from build123d import *

# Parameters (mm, degrees)
SKETCH1_W               = 95.25
SKETCH1_H               = 8.466666667
BOSS_EXTRUDE1_DEPTH     = 38.1
SKETCH2_W               = 6.35
SKETCH2_H               = 127
BOSS_EXTRUDE2_DEPTH     = 38.1
SKETCH3_W               = 88.9
SKETCH3_H               = 8.466666667
BOSS_EXTRUDE3_DEPTH     = 38.1
SKETCH4_R               = 11
CUT_EXTRUDE1_DEPTH      = 149.412147835
SKETCH5_R               = 2.15265
CUT_EXTRUDE2_DEPTH      = 149.412147835
FILLET1_R               = 7.62
BOSS_EXTRUDE4_DEPTH     = 38.1
CUT_EXTRUDE8_REACH      = 172.773
CUT_EXTRUDE8_END_RADIUS = 38.1
FILLET2_R               = 11.688947
FILLET3_R               = 11.688947
FILLET4_R               = 6.35


with BuildPart() as part:
    # Sketch1 → Boss-Extrude1 (new body)
    with BuildSketch(Plane(origin=(0, 0, 0), x_dir=(1, 0, 0), z_dir=(0, 1, 0))):
        with Locations((19.05, 13.758333334)):
            Rectangle(SKETCH1_W, SKETCH1_H)
    extrude(amount=BOSS_EXTRUDE1_DEPTH)

    # Sketch2 → Boss-Extrude2 (add)
    with BuildSketch(Plane(origin=(0, 38.1, 0), x_dir=(1, 0, 0), z_dir=(0, 1, 0))):
        with Locations((63.5, 73.025)):
            Rectangle(SKETCH2_W, SKETCH2_H)
    extrude(amount=-BOSS_EXTRUDE2_DEPTH)

    # Sketch3 → Boss-Extrude3 (add)
    with BuildSketch(Plane(origin=(0, 38.1, 0), x_dir=(1, 0, 0), z_dir=(0, 1, 0))):
        with Locations((15.875, 132.291666667)):
            Rectangle(SKETCH3_W, SKETCH3_H)
    extrude(amount=-BOSS_EXTRUDE3_DEPTH)

    # Sketch4 → Cut-Extrude1 (cut, through all)
    with BuildSketch(Plane(origin=(0, 0, -136.525), x_dir=(-1, 0, 0), z_dir=(0, 0, -1))):
        with Locations((-31.75, 19.05)):
            Circle(SKETCH4_R)
    extrude(amount=-CUT_EXTRUDE1_DEPTH, mode=Mode.SUBTRACT)

    # Sketch5 → Cut-Extrude2 (cut, through all)
    with BuildSketch(Plane(origin=(0, 0, -136.525), x_dir=(-1, 0, 0), z_dir=(0, 0, -1))):
        with Locations((-18.877667779, 26.704865736)):
            Circle(SKETCH5_R)
        with Locations((-19.228536904, 10.833743663)):
            Circle(SKETCH5_R)
        with Locations((-44.622332221, 11.395134264)):
            Circle(SKETCH5_R)
        with Locations((-44.271463096, 27.266256337)):
            Circle(SKETCH5_R)
    extrude(amount=-CUT_EXTRUDE2_DEPTH, mode=Mode.SUBTRACT)

    # Fillet1
    fillet1_edges = [part.edges().sort_by_distance(p)[0] for p in [
        (66.675, 19.05, -136.525),
        (66.675, 19.05, -9.525),
    ]]
    fillet(fillet1_edges, radius=FILLET1_R)

    # Sketch10 → Boss-Extrude4 (add)
    with BuildSketch(Plane(origin=(0, 38.1, 0), x_dir=(1, 0, 0), z_dir=(0, 1, 0))):
        with BuildLine():
            Line((-28.575, 17.991666667), (-28.575, 9.525))
            Line((-28.575, 9.525), (-34.925, 9.525))
            Line((-34.925, 9.525), (-34.925, 25.781))
            Line((-34.925, 25.781), (-5.996027965, 57.15))
            ThreePointArc((-5.996027965, 57.15), (-2.531188929, 73.025), (-5.996027965, 88.9))
            Line((-5.996027965, 88.9), (-34.925, 120.269))
            Line((-34.925, 120.269), (-34.925, 136.525))
            Line((-34.925, 136.525), (-28.575, 136.525))
            Line((-28.575, 136.525), (-28.575, 123.825))
            Line((-28.575, 123.825), (-10.494392478, 104.219375))
            ThreePointArc((-10.494392478, 104.219375), (2.742945437, 73.025), (-10.494392478, 41.830625))
            Line((-10.494392478, 41.830625), (-28.575, 22.225))
            Line((-28.575, 22.225), (-28.575, 17.991666667))
        make_face()
    extrude(amount=-BOSS_EXTRUDE4_DEPTH)

    # Cut-Extrude8: up to this cylinder (the profile starts outside it)
    cut_extrude8_end = Plane(origin=(-40.631188929, 2.695024, -73.025), z_dir=(0, 1, 0)) * Cylinder(CUT_EXTRUDE8_END_RADIUS, 422.746, mode=Mode.PRIVATE)
    # Sketch12 → Cut-Extrude8 (cut, up to the surface)
    with BuildSketch(Plane.ZY.offset(-60.325), mode=Mode.PRIVATE) as cut_extrude8_sk1:
        with BuildLine():
            Line((-79.375, 0), (-66.675, 0))
            ThreePointArc((-66.675, 0), (-73.025, 6.35), (-79.375, 0))
        make_face()
    cut_extrude8_tool1 = extrude(cut_extrude8_sk1.sketch, amount=CUT_EXTRUDE8_REACH, mode=Mode.PRIVATE) - cut_extrude8_end
    add(cut_extrude8_tool1.solids().sort_by_distance((60.325, 2.695024, -73.025))[0], mode=Mode.SUBTRACT)

    # Fillet2
    fillet2_edges = [part.edges().sort_by_distance(p)[0] for p in [
        (-34.925, 19.05, -136.525),
        (-34.925, 19.05, -120.269),
    ]]
    fillet(fillet2_edges, radius=FILLET2_R - 0.0001)  # a hair under: the kernel refuses the full size

    # Fillet3
    fillet3_edges = [part.edges().sort_by_distance(p)[0] for p in [
        (-34.925, 19.05, -25.781),
        (-34.925, 19.05, -9.525),
    ]]
    fillet(fillet3_edges, radius=FILLET3_R - 0.0001)  # a hair under: the kernel refuses the full size

    # Fillet4
    fillet4_edges = [part.edges().sort_by_distance(p)[0] for p in [
        (60.325, 19.05, -17.991666667),
        (60.325, 19.05, -128.058333333),
    ]]
    fillet(fillet4_edges, radius=FILLET4_R)


solid = part.part
Geometry: final body of the model. Coordinates: model frame, mm. A direction names the side the tool comes from. Coordinates: 2 decimals unless noted, no trailing zeros. Loops run counter-clockwise (first coordinate to the right, second up) from the corner with the lowest first, then second, coordinate; pieces in that order, holes last. Notation, with made-up numbers: (28.25, 46) - (33.25, 46) arc R13 cw to (33.25, 65) - close; hole circle Ø10 at (24.25, -13). An arc over 180 degrees is marked (long way). Put each result on its own line as item: value. Start each with the question number.
Q1. Cut plane A-A, the plane x = 31.75. Return loops of the section in (y, z) (3 decimals), and give its area (3 significant figures).
Q2. Line query: line 1 (Z direction, x = 44, y = 20) (3 decimals); line 2 (Z direction, x = -23, y = 29.5) (3 decimals); line 3 (Y direction, x = 31.75, z = -131). Output: solid intervals per line, ascending.
Q3. Set-up query: faces 4 (the flat face through (-28.575, 19, -126)), 5 (the flat face through (-19, 19, -103)), 6 (the cylindrical face through (45.86, 28.72, -132.35)). Return all of +Z, -Z, +X, -X, +Y, -Y with unobstructed straight access to the full face (end or side cutting, diameter ignored); none if empty.
Q4. Pin query (flat end, axial travel): pin 1 Ø1 at (y, z) = (4, -37) entering from -X; pin 2 Ø1.5 at (y, z) = (18, -101) entering from -X. Return the tip coordinate at first contact, or that it passes through.
Q5. Cut plane C-C, the plane z = -84.5. Return loops of the section in (x, y) (1 decimal), and give its area (3 significant figures).
Q6. Pull-direction query (Z, two-part tool) for faces 1 (the cylindrical face through (45.86, 28.72, -13.82)), 2 (the flat face through (12, 19, -128.058)), 3 (the cylindrical face through (64.384, 18.783, -134.352)); classes: released by +Z, released by -Z, zero draft, split by the parting line, or undercut.
Filled sheet:
1. outline: (0, -136.525) - (8.05, -136.525) - (8.05, -128.058) - (0, -128.058) - close; (0, -17.992) - (8.05, -17.992) - (8.05, -9.525) - (0, -9.525) - close; (30.05, -136.525) - (38.1, -136.525) - (38.1, -128.058) - (30.05, -128.058) - close; (30.05, -17.992) - (38.1, -17.992) - (38.1, -9.525) - (30.05, -9.525) - close
1. area: 273 mm²
2. line 1: -136.525 to -128.058, -17.992 to -9.525
2. line 2: -136.525 to -128.058, -117.78 to -107.338, -38.712 to -28.27, -17.992 to -9.525
2. line 3: 0 to 8.05, 30.05 to 38.1
3. face 4: +Y, -Y
3. face 5: -X, +Y, -Y
3. face 6: +Z, -Z
4. pin 1: x = -25.04
4. pin 2: x = -17.85
5. outline: (-4.3, 0) - (1.2, 0) - (1.2, 38.1) - (-4.3, 38.1) - close; (60.3, 0) - (66.7, 0) - (66.7, 38.1) - (60.3, 38.1) - close
5. area: 451 mm²
6. face 1: zero draft
6. face 2: undercut
6. face 3: released by -Z
